Can you work these out from the model? Positions are in its coordinate system, mm. Give positions to 0.01 mm unless a question says otherwise; leave off trailing zeros. Answer as a JSON object with one key per item and string values.
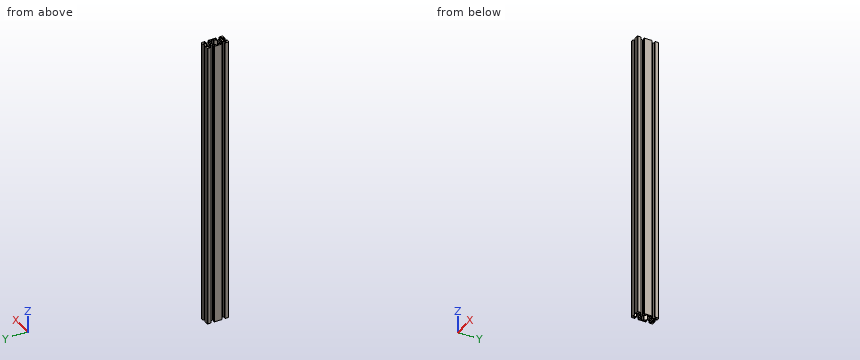
Autodesk Inventor part; units mm, degrees
ref_plane "C1_XY" through (0, 0, 0) normal (0, 0, 1) x (1, 0, 0)
ref_plane "C1_YZ" through (0, 0, 0) normal (1, 0, 0) x (0, 1, 0)
ref_plane "C1_ZX" through (0, 0, 0) normal (0, 1, 0) x (0, 0, 1)
sketch "Sketch_1" plane through (0, 0, 0) normal (0, 0, 1) x (1, 0, 0)
  line L0 (-10, -7) -> (-8, -7)
  line L1 (-8, -7) -> (-8, -4)
  line L2 (-8, -4) -> (-7.0607, -4)
  line L3 (-7.0607, -4) -> (-4, -7.0607)
  line L4 (-4, -7.0607) -> (-4, -9.4804)
  line L5 (-4, -9.4804) -> (-3.7, -10)
  line L6 (-3.7, -10) -> (-4, -10.5196)
  line L7 (-4, -10.5196) -> (-4, -12.9393)
  line L8 (-4, -12.9393) -> (-7.0607, -16)
  line L9 (-7.0607, -16) -> (-8, -16)
  line L10 (-8, -16) -> (-8, -13)
  line L11 (-8, -13) -> (-10, -13)
  line L12 (-10, -13) -> (-10, -19)
  arc A0 (-10, -19) -> (-9, -20) centre (-9, -19) ccw
  line L13 (-9, -20) -> (-3, -20)
  line L14 (-3, -20) -> (-3, -18)
  line L15 (-3, -18) -> (-6, -18)
  line L16 (-6, -18) -> (-6, -17.0607)
  line L17 (-6, -17.0607) -> (-2.9393, -14)
  line L18 (-2.9393, -14) -> (-0.5196, -14)
  line L19 (-0.5196, -14) -> (0, -13.7)
  line L20 (0, -13.7) -> (0.5196, -14)
  line L21 (0.5196, -14) -> (2.9393, -14)
  line L22 (2.9393, -14) -> (6, -17.0607)
  line L23 (6, -17.0607) -> (6, -18)
  line L24 (6, -18) -> (3, -18)
  line L25 (3, -18) -> (3, -20)
  line L26 (3, -20) -> (9, -20)
  arc A1 (9, -20) -> (10, -19) centre (9, -19) ccw
  line L27 (10, -19) -> (10, -13)
  line L28 (10, -13) -> (8, -13)
  line L29 (8, -13) -> (8, -16)
  line L30 (8, -16) -> (7.0607, -16)
  line L31 (7.0607, -16) -> (4, -12.9393)
  line L32 (4, -12.9393) -> (4, -10.5196)
  line L33 (4, -10.5196) -> (3.7, -10)
  line L34 (3.7, -10) -> (4, -9.4804)
  line L35 (4, -9.4804) -> (4, -7.0607)
  line L36 (4, -7.0607) -> (7.0607, -4)
  line L37 (7.0607, -4) -> (8, -4)
  line L38 (8, -4) -> (8, -7)
  line L39 (8, -7) -> (10, -7)
  line L40 (10, -7) -> (10, 7)
  line L41 (10, 7) -> (8, 7)
  line L42 (8, 7) -> (8, 4)
  line L43 (8, 4) -> (7.0607, 4)
  line L44 (7.0607, 4) -> (4, 7.0607)
  line L45 (4, 7.0607) -> (4, 9.4804)
  line L46 (4, 9.4804) -> (3.7, 10)
  line L47 (3.7, 10) -> (4, 10.5196)
  line L48 (4, 10.5196) -> (4, 12.9393)
  line L49 (4, 12.9393) -> (7.0607, 16)
  line L50 (7.0607, 16) -> (8, 16)
  line L51 (8, 16) -> (8, 13)
  line L52 (8, 13) -> (10, 13)
  line L53 (10, 13) -> (10, 19)
  arc A2 (10, 19) -> (9, 20) centre (9, 19) ccw
  line L54 (9, 20) -> (3, 20)
  line L55 (3, 20) -> (3, 18)
  line L56 (3, 18) -> (6, 18)
  line L57 (6, 18) -> (6, 17.0607)
  line L58 (6, 17.0607) -> (2.9393, 14)
  line L59 (2.9393, 14) -> (0.5196, 14)
  line L60 (0.5196, 14) -> (0, 13.7)
  line L61 (0, 13.7) -> (-0.5196, 14)
  line L62 (-0.5196, 14) -> (-2.9393, 14)
  line L63 (-2.9393, 14) -> (-6, 17.0607)
  line L64 (-6, 17.0607) -> (-6, 18)
  line L65 (-6, 18) -> (-3, 18)
  line L66 (-3, 18) -> (-3, 20)
  line L67 (-3, 20) -> (-9, 20)
  arc A3 (-9, 20) -> (-10, 19) centre (-9, 19) ccw
  line L68 (-10, 19) -> (-10, 13)
  line L69 (-10, 13) -> (-8, 13)
  line L70 (-8, 13) -> (-8, 16)
  line L71 (-8, 16) -> (-7.0607, 16)
  line L72 (-7.0607, 16) -> (-4, 12.9393)
  line L73 (-4, 12.9393) -> (-4, 10.5196)
  line L74 (-4, 10.5196) -> (-3.7, 10)
  line L75 (-3.7, 10) -> (-4, 9.4804)
  line L76 (-4, 9.4804) -> (-4, 7.0607)
  line L77 (-4, 7.0607) -> (-7.0607, 4)
  line L78 (-7.0607, 4) -> (-8, 4)
  line L79 (-8, 4) -> (-8, 7)
  line L80 (-8, 7) -> (-10, 7)
  line L81 (-10, 7) -> (-10, -7)
  line L82 (-8, 1.7) -> (-8, -1.7)
  arc A4 (-8, -1.7) -> (-7.7, -2) centre (-7.7, -1.7) ccw
  line L83 (-7.7, -2) -> (-7.0636, -2)
  arc A5 (-6.8515, -2.0879) -> (-7.0636, -2) centre (-7.0636, -2.3) ccw
  line L84 (-6.8515, -2.0879) -> (-2.9393, -6)
  line L85 (-2.9393, -6) -> (2.9393, -6)
  line L86 (2.9393, -6) -> (6.8515, -2.0879)
  arc A6 (7.0636, -2) -> (6.8515, -2.0879) centre (7.0636, -2.3) ccw
  line L87 (7.0636, -2) -> (7.7, -2)
  arc A7 (7.7, -2) -> (8, -1.7) centre (7.7, -1.7) ccw
  line L88 (8, -1.7) -> (8, 1.7)
  arc A8 (8, 1.7) -> (7.7, 2) centre (7.7, 1.7) ccw
  line L89 (7.7, 2) -> (7.0636, 2)
  arc A9 (6.8515, 2.0879) -> (7.0636, 2) centre (7.0636, 2.3) ccw
  line L90 (6.8515, 2.0879) -> (2.9393, 6)
  line L91 (2.9393, 6) -> (-2.9393, 6)
  line L92 (-2.9393, 6) -> (-6.8515, 2.0879)
  arc A10 (-7.0636, 2) -> (-6.8515, 2.0879) centre (-7.0636, 2.3) ccw
  line L93 (-7.0636, 2) -> (-7.7, 2)
  arc A11 (-7.7, 2) -> (-8, 1.7) centre (-7.7, 1.7) ccw
extrude "Extrusion1" add sketch "Sketch_1" against normal blind 530
sketch "Sketch2" plane through (0, 0, -530) normal (0, 0, -1) x (-1, 0, 0)
  point P0 (0, 10)
hole "Hole1" at (0, 10, -530) direction (0, 0, 1) diameter 4.2 depth 530
pattern_linear "Rectangular Pattern1" count 2 spacing 20 along (0, -1, 0) of "Hole1"
ref_plane "C1_XY" through (0, 0, 0) normal (0, 0, 1) x (1, 0, 0)
ref_plane "C1_YZ" through (0, 0, 0) normal (1, 0, 0) x (0, 1, 0)
ref_plane "C1_ZX" through (0, 0, 0) normal (0, 1, 0) x (0, 0, 1)
properties part number "HFS5-2040-530"
1) I need wall thicknesses on L1, parallel to Y at x = 0.5, z = -130; L2, parallel to Y at x = 0, z = -168.5; L3, parallel to X at y = 0, z = -124.5. Which ranges of each line are inside material? Lowest first, please.
Check sheet entries:
{"L1": "-13.99 to -12.04, -7.96 to -6, 6 to 7.96, 12.04 to 13.99", "L2": "-13.7 to -12.1, -7.9 to -6, 6 to 7.9, 12.1 to 13.7", "L3": "-10 to -8, 8 to 10"}
2) I'm going to push flat-ended pins straight in: P1, Ø1, axis at x = 2, z = -60, coming from the -Y side; P2, Ø3, axis at x = 0, z = -304.5, coming from the +Y side. Where does each tip first touch, or does it pass through?
Check sheet entries:
{"P1": "y = -14", "P2": "y = 14"}
3) Imagine slicing it at A-A on z = -44. Give the number of separate pieces and of enclosed holes in the cut face, and give its area (3 significant figures).
Check sheet entries:
{"separate pieces": "1", "enclosed holes": "3", "area": "324 mm2"}
